Verification items for this drawing (mm, ordinates from the low corner). A direction names the side the tool comes from. Give positions to 0.01 mm unless a question says otherwise; leave off trailing zeros. Write each loop counter-clockwise with the first axis right and the second up, starting at its lowest first coordinate (ties: lowest second). Pieces come first, ordered by that corner, then holes. Notation, with made-up numbers: (-27, 43) -> (27, 43) arc R8 ccw to (27, 56) -> close; hole circle Ø6 at (2, 42). An arc over 180 degrees is marked (long way). Answer as a JSON object with one key per item and string values.
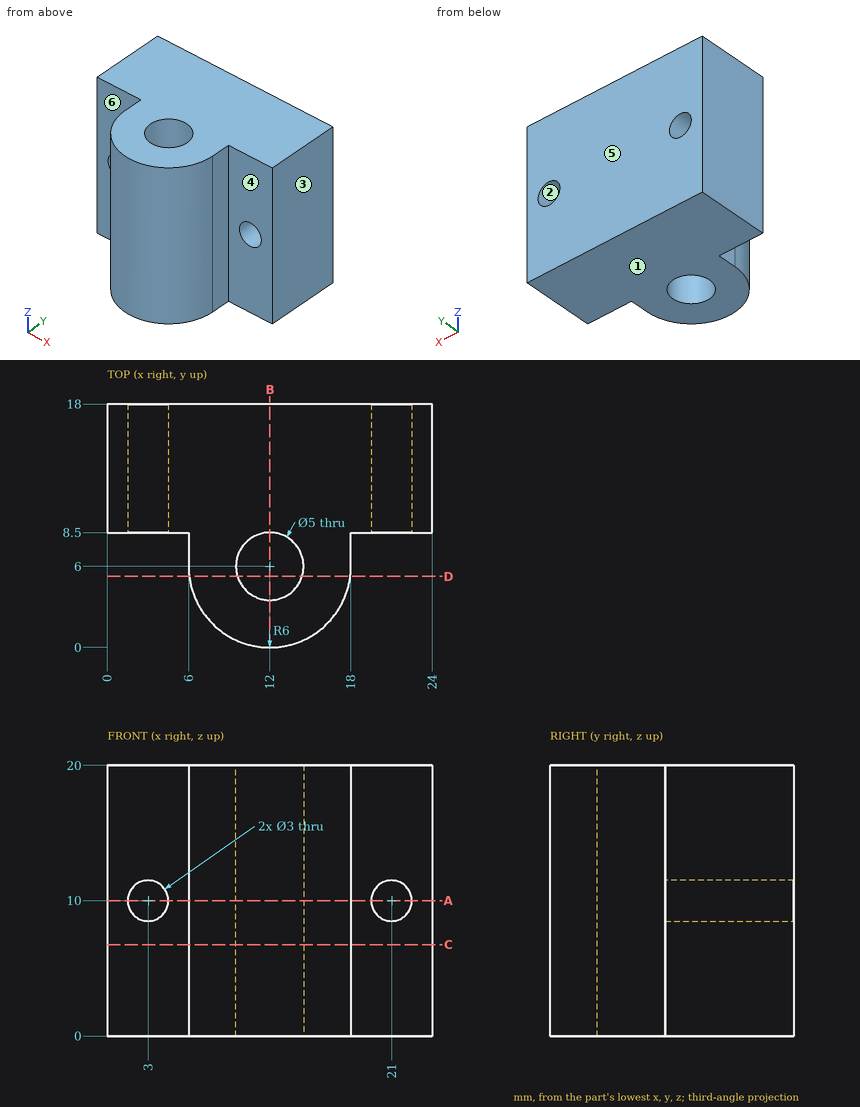
1. Sectioned sample at A-A, the plane z = 10. Enter the section's corners in (x, y).
Determined:
{"outline": "(0, 8.5) -> (1.5, 8.5) -> (1.5, 18) -> (0, 18) -> close; (4.5, 8.5) -> (6, 8.5) -> (6, 6) arc R6 ccw to (18, 6) -> (18, 8.5) -> (19.5, 8.5) -> (19.5, 18) -> (4.5, 18) -> close; (22.5, 8.5) -> (24, 8.5) -> (24, 18) -> (22.5, 18) -> close; hole circle Ø5 at (12, 6)"}
2. Access from +Z, -Z, +X, -X, +Y, -Y to the whole of each face (thin tool, end or side, straight path). Record for the marked faces 4, 5 and 6.
Determined:
{"face 4": "+Z, -Z, +X, -Y", "face 5": "+Z, -Z, +X, -X, +Y", "face 6": "+Z, -Z, -X, -Y"}
3. Sectioned sample at C-C, the plane z = 6.75. Enter the section's corners in (x, y), plus the area to 3 significant figures.
Determined:
{"outline": "(0, 8.5) -> (6, 8.5) -> (6, 6) arc R6 ccw to (18, 6) -> (18, 8.5) -> (24, 8.5) -> (24, 18) -> (0, 18) -> close; hole circle Ø5 at (12, 6)", "area": "295 mm^2"}
4. Go/stop test with flat-tipped pins: P1, Ø3, axis at x = 7.5, z = 13, coming from the -Y side; P2, Ø1.8, axis at x = 2.5, z = 12.5, coming from the -Y side; P3, Ø1.2, axis at y = 7, z = 8, coming from the -X side. Record where each tip stops, or that it passes through.
Determined:
{"P1": "y = 0.8", "P2": "y = 8.5", "P3": "x = 6"}
5. Scan lines: L1, parallel to X at y = 15.25, z = 10; L2, parallel to Y at x = 12, z = 15.25; L3, parallel to X at y = 9, z = 11. Record each from-to range of solid material in increasing order. Write a range as [from, to].
Determined:
{"L1": "[0, 1.5], [4.5, 19.5], [22.5, 24]", "L2": "[0, 3.5], [8.5, 18]", "L3": "[0, 1.88], [4.12, 19.88], [22.12, 24]"}
6. Mould release check, pull along X, two halves, no side actions. Record for the marked faces 1, 2 and 3: released by +X, released by -X, zero draft, split by the parting line, or undercut.
Determined:
{"face 1": "zero draft", "face 2": "undercut", "face 3": "released by +X"}
7. Sectioned sample at B-B, the plane x = 12. Enter the section's corners in (y, z).
Determined:
{"outline": "(0, 0) -> (3.5, 0) -> (3.5, 20) -> (0, 20) -> close; (8.5, 0) -> (18, 0) -> (18, 20) -> (8.5, 20) -> close"}
8. Sectioned sample at D-D, the plane y = 5.25. Enter the section's corners in (x, z), plus the area to 3 significant figures.
Determined:
{"outline": "(6.05, 0) -> (9.62, 0) -> (9.62, 20) -> (6.05, 20) -> close; (14.38, 0) -> (17.95, 0) -> (17.95, 20) -> (14.38, 20) -> close", "area": "143 mm^2"}
